Answer from the drawing. Dimensions are ordinates in mm from the lowest x, y and z of the part. A direction names the side the tool comes from. Coordinates: 2 decimals unless noted, no trailing zeros. Write each loop counter-clockwise with the first axis right and the second up, starting at its lowest first coordinate (ties: lowest second). Pieces come first, ordered by that corner, then holes. Notation, with made-up numbers: (23.5, 28.5) - (80.5, 28.5) arc R25 ccw to (80.5, 44.5) - close; hole circle Ø9 at (22, 3). An arc over 180 degrees is marked (long way). Return JSON: item names as keys, results as strings.
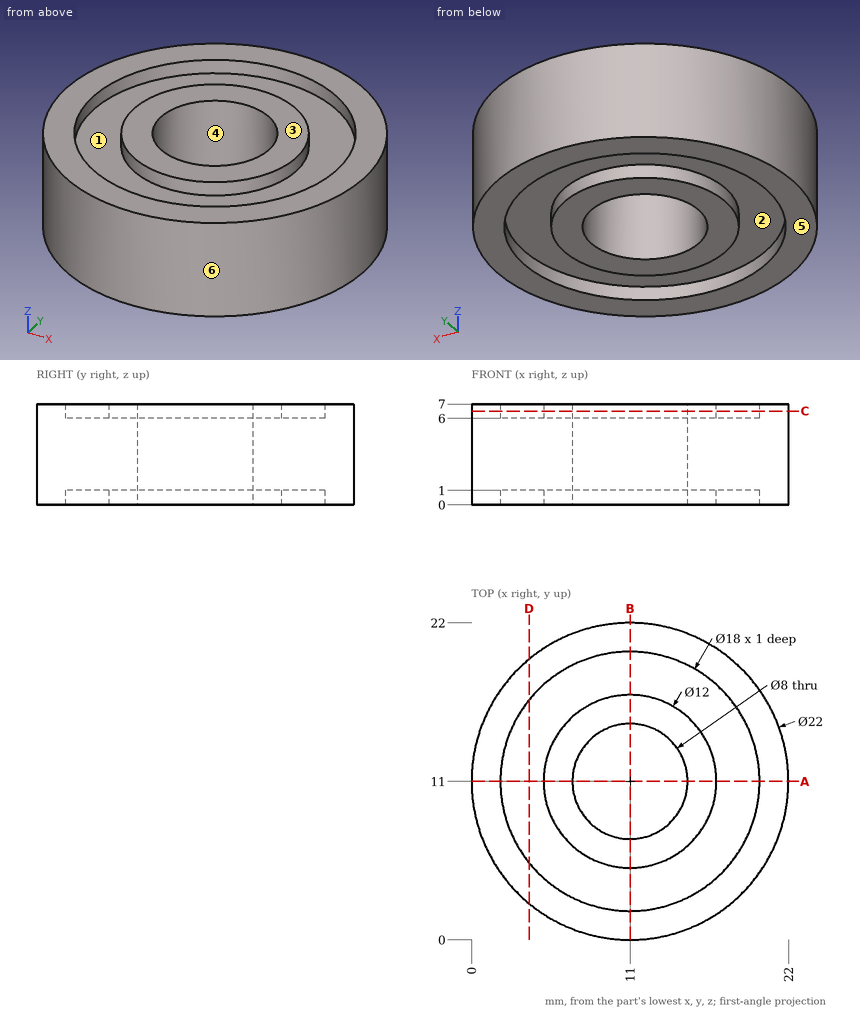
(1) A cutting plane is placed at D-D (x = 4). Determine the outline of the cut face in (y, z), and give its area (3 significant figures).
Answer:
{"outline": "(2.51, 0) - (5.34, 0) - (5.34, 1) - (16.66, 1) - (16.66, 0) - (19.49, 0) - (19.49, 7) - (16.66, 7) - (16.66, 6) - (5.34, 6) - (5.34, 7) - (2.51, 7) - close", "area": "96.2 mm²"}
(2) A cutting plane is placed at A-A (y = 11). Determine the outline of the cut face in (x, z), and give its area (3 significant figures).
Answer:
{"outline": "(0, 0) - (2, 0) - (2, 1) - (5, 1) - (5, 0) - (7, 0) - (7, 7) - (5, 7) - (5, 6) - (2, 6) - (2, 7) - (0, 7) - close; (15, 0) - (17, 0) - (17, 1) - (20, 1) - (20, 0) - (22, 0) - (22, 7) - (20, 7) - (20, 6) - (17, 6) - (17, 7) - (15, 7) - close", "area": "86.0 mm²"}
(3) A cutting plane is placed at C-C (z = 6.5). Determine the outline of the cut face in (x, y), and give its area (3 significant figures).
Answer:
{"outline": "circle Ø22 at (11, 11); circle Ø12 at (11, 11); hole circle Ø18 at (11, 11); hole circle Ø8 at (11, 11)", "area": "188 mm²"}
(4) Straight lines are drawn through the part: line 1 (Y direction, x = 11, z = 6.45); line 2 (Y direction, x = 11, z = 2.25); line 3 (Y direction, x = 9.5, z = 1.5). For each, find the intervals that lie inside material, in ascending order. Write a range as from..to.
Answer:
{"line 1": "0..2, 5..7, 15..17, 20..22", "line 2": "0..7, 15..22", "line 3": "0.1..7.29, 14.71..21.9"}
(5) Flat-ended cylindrical pins translate along their axes: P1, Ø6.5, axis at x = 11, y = 11, coming from the +Z side (3 decimals); P2, Ø4, axis at y = 17.5, z = 1, coming from the +X side. Find the tip coordinate at first contact, or state that the pin passes through.
Answer:
{"P1": "through", "P2": "x = 21.04"}
(6) Determine the mould class of the marked faces 4, 5 and 6 for opening direction Y: +Y half, -Y half, draft (parallel to the pull), parting line (faces both ways), or undercut.
Answer:
{"face 4": "undercut", "face 5": "draft", "face 6": "parting line"}
(7) Which of the six approach directions +Z, -Z, +X, -X, +Y, -Y give full straight-line access (tool end or side, diameter ignored) to the marked faces 1, 2 and 3?
Answer:
{"face 1": "+Z", "face 2": "-Z", "face 3": "+Z, +X, -X, +Y, -Y"}
